```python
from build123d import *

# Parameters (mm, degrees)
BOSS_EXTRUDE1_DEPTH = 2
EDGE_FLANGE1_DEPTH  = 2
EDGE_FLANGE2_DEPTH  = 2
SKETCH13_W          = 2.5
SKETCH13_H          = 2.15
SKETCH13_W_2        = 3
CUT_EXTRUDE3_DEPTH  = 10


# Sheet-metal steps are written as plain solids
with BuildPart() as part:
    # Sketch2 → Boss-Extrude1 (new body)
    with BuildSketch(Plane(origin=(0, 0, 0), x_dir=(1, 0, 0), z_dir=(0, 1, 0))):
        Polygon((-52.543309772, 32.413356753), (-54.793309772, 32.413356753), (-54.793309772, 30.413356753), (64.413548219, 30.413356753), (67.959993108, 26.866911863), (67.959993108, 23.966910068), (75.359993548, 16.566912168), (75.359993548, -11.849150158), (67.759993508, -19.449150198), (67.759993508, -31.745752353), (62.750836838, -36.754909023), (58.359994528, -36.754909023), (58.359994528, -42.739906444), (71.753176861, -42.739906444), (75.659994488, -38.833088817), (75.659994488, -22.433088597), (81.359993248, -16.733089837), (81.359993248, 1.669814581), (83.609993248, 1.669814581), (83.609993248, 3.669814581), (81.359993248, 3.669814581), (81.359993248, 19.459804242), (66.106440177, 34.713357313), (-52.543309772, 34.713357313), align=None)
    extrude(amount=BOSS_EXTRUDE1_DEPTH)

    # Edge-Flange1 section (across the edge) → Edge-Flange1 (add)
    with BuildSketch(Plane(origin=(-55.793309772, 0, -30.413356753), x_dir=(1, 0, 0), z_dir=(0, 0, -1))):
        with BuildLine():
            Line((-2, 0.5), (-2, 11.4))
            Line((-2, 11.4), (0, 11.4))
            Line((0, 11.4), (0, 0.5))
            ThreePointArc((0, 0.5), (0.146446609, 0.146446609), (0.5, 0))
            Line((0.5, 0), (1, 0))
            Line((1, 0), (1, -2))
            Line((1, -2), (0.5, -2))
            ThreePointArc((0.5, -2), (-1.267766953, -1.267766953), (-2, 0.5))
        make_face()
    extrude(amount=EDGE_FLANGE1_DEPTH)

    # Edge-Flange2 section (across the edge) → Edge-Flange2 (add)
    with BuildSketch(Plane(origin=(84.609993248, 0, -3.669814581), x_dir=(-1, 0, 0), z_dir=(0, 0, 1))):
        with BuildLine():
            Line((-2, 0.5), (-2, 11.4))
            Line((-2, 11.4), (0, 11.4))
            Line((0, 11.4), (0, 0.5))
            ThreePointArc((0, 0.5), (0.146446609, 0.146446609), (0.5, 0))
            Line((0.5, 0), (1, 0))
            Line((1, 0), (1, -2))
            Line((1, -2), (0.5, -2))
            ThreePointArc((0.5, -2), (-1.267766953, -1.267766953), (-2, 0.5))
        make_face()
    extrude(amount=EDGE_FLANGE2_DEPTH)

    # Sketch13 → Cut-Extrude3 (cut)
    with BuildSketch(Plane(origin=(0, 2, 0), x_dir=(1, 0, 0), z_dir=(0, 1, 0))):
        with Locations((-27.730006168, 34.839358373)):
            Rectangle(SKETCH13_W, SKETCH13_H)
        with Locations((-41.672006168, 34.839358373)):
            Rectangle(SKETCH13_W_2, SKETCH13_H)
        with Locations((-12.490006168, 34.839358373)):
            Rectangle(SKETCH13_W, SKETCH13_H)
        with Locations((2.749993832, 34.839358373)):
            Rectangle(SKETCH13_W, SKETCH13_H)
        with Locations((17.608993832, 34.839358373)):
            Rectangle(SKETCH13_W, SKETCH13_H)
        with Locations((32.213993832, 34.839358373)):
            Rectangle(SKETCH13_W, SKETCH13_H)
        with Locations((47.453993832, 34.839358373)):
            Rectangle(SKETCH13_W, SKETCH13_H)
        with Locations((61.931993832, 34.839358373)):
            Rectangle(SKETCH13_W, SKETCH13_H)
    extrude(amount=-CUT_EXTRUDE3_DEPTH, mode=Mode.SUBTRACT)


solid = part.part
```
Can you work these out from the model? Positions are in its coordinate system, mm. A direction names the side the tool comes from. Round coordinates to 2 decimals unless told otherwise and drop trailing zeros. Order: outer loops, then holes, each group sorted by start corner. A loop starts at its lowest first (then second) coordinate and runs counter-clockwise, first axis right, second up. Notation, with made-up numbers: (52.25, 26) -> (57.25, 26) arc R18 cw to (57.25, 59) -> close; hole circle Ø3 at (62, -8). An arc over 180 degrees is marked (long way). Return JSON: item names as keys, results as strings. Group by question number.
1. We'd pull the mould along Z, two halves only. Please class faces 6 (the face through (-56, -3, -32.413)), 7 (the face through (71.61, 0.99, 15.6)), 8 (the face through (73.679, 0.986, 40.814)): released by +Z, released by -Z, zero draft, split by the parting line, or undercut.
2. If we section it at A-A, the plane y = -5: Write out the boundary of the cut face in (x, z).
3. If we section it at B-B, the plane x = 69.5: Write out the boundary of the cut face in (y, z), then the cut area to 3 significant figures.
4. I need wall thicknesses on line 1 (X direction, y = 1.5, z = -10.5); line 2 (X direction, y = 0.75, z = -24). Which ranges of each line are inside material? Lowest first, please. Write a range as [from, to].
5. Which directions (+Z, -Z, +X, -X, +Y, -Y) give clear straight access to the entire face, cutting with the end or side of a thin tool? Please do faces 1 (the face through (85, -3, -1.67)), 2 (the face through (71.608, 0.986, -20.319)), 3 (the face through (-57.04, 1.29, -31.4)), 4 (the face through (85, -3, -3.67)), 5 (the face through (85.858, 1.287, -2.684)).
6. If we section it at D-D, the plane z = 30: Write out the boundary of the cut face in (x, y).
7. If we section it at C-C, the plane z = 6.5: Write out the boundary of the cut face in (x, y), then the cut area to 3 significant figures.
8. Will these pins go through, and if not, where does the flat tip stop? pin 1 (6 mm diameter, centred on y = 0.5, z = -8.5, fed in from +X); pin 2 (0.6 mm diameter, centred on y = 1.5, z = 31.5, fed in from +X); pin 3 (0.8 mm diameter, centred on y = 1, z = -34, fed in from +X); pin 4 (5 mm diameter, centred on y = -3.5, z = 31, fed in from -X).
Output values:
{
 "1": {"face 6": "released by -Z", "face 7": "undercut", "face 8": "released by +Z"},
 "2": {"outline": "(-57.79, -32.41) -> (-55.79, -32.41) -> (-55.79, -30.41) -> (-57.79, -30.41) -> close; (84.61, -3.67) -> (86.61, -3.67) -> (86.61, -1.67) -> (84.61, -1.67) -> close"},
 "3": {"outline": "(0, -31.32) -> (2, -31.32) -> (2, -22.43) -> (0, -22.43) -> close; (0, 17.71) -> (2, 17.71) -> (2, 42.74) -> (0, 42.74) -> close", "area": "67.8 mm²"},
 "4": {"line 1": "[75.36, 81.36]", "line 2": "[67.96, 76.82]"},
 "5": {"face 1": "+Z, +X, +Y, -Y", "face 2": "-X, +Y, -Y", "face 3": "+Z, -Z, -X, +Y", "face 4": "-Z, +X, +Y, -Y", "face 5": "+Z, -Z, +X, +Y"},
 "6": {"outline": "(67.76, 0) -> (75.66, 0) -> (75.66, 2) -> (67.76, 2) -> close"},
 "7": {"outline": "(75.36, 0) -> (81.36, 0) -> (81.36, 2) -> (75.36, 2) -> close", "area": "12.0 mm²"},
 "8": {"pin 1": "x = 81.36", "pin 2": "x = 75.66", "pin 3": "x = 67.22", "pin 4": "through"}
}
